```python
from build123d import *

# Parameters (mm, degrees)
F1_DEPTH = 17.5
F2_DEPTH = 2.8
F4_DEPTH = 2.8
F6_DEPTH = 2.8


with BuildPart() as f1:
    # F0 (on Front) → F1 (new body)
    with BuildSketch(Plane.XZ):
        Polygon((0, 37.5), (0, 0), (37.5, 0), (37.5, 2.8), (2.8, 2.8), (2.8, 37.5), align=None)
    extrude(amount=F1_DEPTH)

    # F0 (on Front) → F2 (join)
    with BuildSketch(Plane.XZ):
        Polygon((2.8, 2.8), (37.5, 2.8), (37.5, 3), (3, 37.5), (2.8, 37.5), align=None)
    extrude(amount=F2_DEPTH)

    # F3 (on face) → F4 (cut, through all)
    with BuildSketch(Plane(origin=(0, 0, 0), x_dir=(0, -1, 0), z_dir=(-1, 0, 0))):
        with BuildLine():
            ThreePointArc((11.5, 31.4665), (8.75, 33.20004), (6, 31.4665))
            Line((6, 31.4665), (6, 25.5335))
            ThreePointArc((6, 25.5335), (8.75, 23.79996), (11.5, 25.5335))
            Line((11.5, 25.5335), (11.5, 31.4665))
        make_face()
        with BuildLine():
            ThreePointArc((11.5, 14.0665), (8.75, 15.80004), (6, 14.0665))
            Line((6, 14.0665), (6, 8.1335))
            ThreePointArc((6, 8.1335), (8.75, 6.39996), (11.5, 8.1335))
            Line((11.5, 8.1335), (11.5, 14.0665))
        make_face()
    extrude(amount=-F4_DEPTH, mode=Mode.SUBTRACT)

    # F5 (on face) → F6 (cut, through all)
    with BuildSketch(Plane(origin=(0, 0, 0), x_dir=(1, 0, 0), z_dir=(0, 0, -1))):
        with BuildLine():
            ThreePointArc((25.5335, 11.5), (23.79996, 8.75), (25.5335, 6))
            Line((25.5335, 6), (31.4665, 6))
            ThreePointArc((31.4665, 6), (33.20004, 8.75), (31.4665, 11.5))
            Line((31.4665, 11.5), (25.5335, 11.5))
        make_face()
        with BuildLine():
            ThreePointArc((8.1335, 11.5), (6.39996, 8.75), (8.1335, 6))
            Line((8.1335, 6), (14.0665, 6))
            ThreePointArc((14.0665, 6), (15.80004, 8.75), (14.0665, 11.5))
            Line((14.0665, 11.5), (8.1335, 11.5))
        make_face()
    extrude(amount=-F6_DEPTH, mode=Mode.SUBTRACT)


solid = f1.part
```
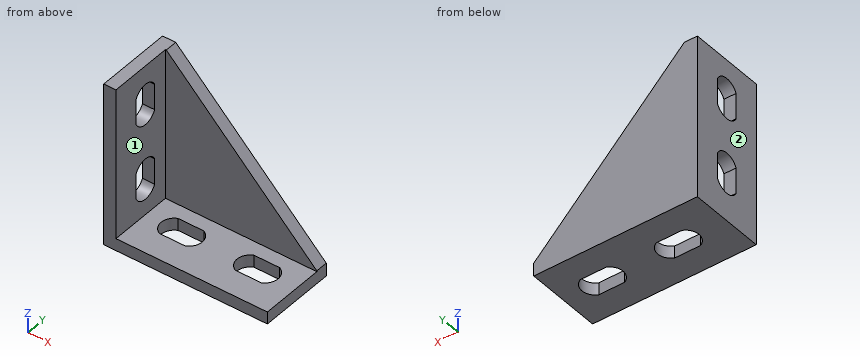
For this review, take the finished solid that the model builds, in its own axes (mm). Face numbers are marked on the shaded views. A direction names the side the tool comes from. Round coordinates to 2 decimals unless told otherwise and drop trailing zeros. Write each loop counter-clockwise with the first axis right and the second up, starting at its lowest first coordinate (ties: lowest second). Pieces come first, ordered by that corner, then holes. Notation, with made-up numbers: (37, 25) -> (68, 25) arc R23 cw to (68, 50) -> close; hole circle Ø3 at (47, -16.75). An arc over 180 degrees is marked (long way). One line per question, with ' | ' between items. Start each with the question number.
(1) For line 1 along Z through (x, y) = (17, -11); line 2 along Y through (x, z) = (22.5, 9), list the stretches that pass through material, from the lowest coordinate up. Write a range as from..to.
(2) Add section C-C, the plane y = -8.5. Write out the cut boundary in (x, z), plus the area to 3 significant figures.
(3) Tool access review of the marked faces 1 and 2: name each direction out of +Z, -Z, +X, -X, +Y, -Y from which nothing blocks a thin tool from reaching the whole face with its end or side.
(4) Add section B-B, the plane x = 11. Write out the cut boundary in (y, z), plus the area to 3 significant figures.
(5) Add section A-A, the plane z = 13. Write out the cut boundary in (x, y).
(6) Add section D-D, the plane x = 17.5. Write out the cut boundary in (y, z).
(7) Insertion check: P1, Ø0.8, axis at x = 9.5, z = 2, coming from the +Y side; P2, Ø8, axis at x = 28.5, z = 15, coming from the -Y side; P3, Ø1.5, axis at x = 22.5, y = -12, coming from the +Z side. Each pin has a flat end and moves straight along its axis. Give the tip position at first contact, or say it passes through.
Answer list:
1) line 1: 0..2.8 | line 2: -2.8..0
2) outline: (0, 0) -> (6.41, 0) -> (6.41, 2.8) -> (2.8, 2.8) -> (2.8, 6.41) -> (0, 6.41) -> close; (0, 15.79) -> (2.8, 15.79) -> (2.8, 23.81) -> (0, 23.81) -> close; (0, 33.19) -> (2.8, 33.19) -> (2.8, 37.5) -> (0, 37.5) -> close; (15.79, 0) -> (23.81, 0) -> (23.81, 2.8) -> (15.79, 2.8) -> close; (33.19, 0) -> (37.5, 0) -> (37.5, 2.8) -> (33.19, 2.8) -> close | area: 97.1 mm²
3) face 1: +Z, +X, -Y | face 2: +Z, -Z, -X, +Y, -Y
4) outline: (-17.5, 0) -> (-11.5, 0) -> (-11.5, 2.8) -> (-17.5, 2.8) -> close; (-6, 0) -> (0, 0) -> (0, 29.5) -> (-2.8, 29.5) -> (-2.8, 2.8) -> (-6, 2.8) -> close | area: 108 mm²
5) outline: (0, -17.5) -> (2.8, -17.5) -> (2.8, -11.5) -> (0, -11.5) -> close; (0, -6) -> (2.8, -6) -> (2.8, -2.8) -> (27.5, -2.8) -> (27.5, 0) -> (0, 0) -> close
6) outline: (-17.5, 0) -> (0, 0) -> (0, 23) -> (-2.8, 23) -> (-2.8, 2.8) -> (-17.5, 2.8) -> close
7) P1: y = 0 | P2: y = -2.8 | P3: z = 2.8
